Build history of the part. All positions in model axes, mm. Face numbers are marked on the shaded views. Round coordinates to 2 decimals unless told otherwise and drop trailing zeros. Loops run counter-clockwise (first coordinate to the right, second up) from the corner with the lowest first, then second, coordinate; pieces in that order, holes last. Notation, with made-up numbers: (23.25, -35) - (52.25, -35) arc R17 cw to (52.25, -9) - close; hole circle Ø5 at (36, -15.75). An arc over 180 degrees is marked (long way). Put each result on its own line as item: value. Start each with the question number.
from build123d import *

# Parameters (mm, degrees)
SKETCH1_W                      = 600
SKETCH1_H                      = 206.35
BASE_FLANGE1_DEPTH             = 3.18
SKETCH6_W                      = 25.4
SKETCH6_H                      = 6
CUT_EXTRUDE1_DEPTH             = 10
EDGE_FLANGE1_STRIP_W           = 14.1932
EDGE_FLANGE1_STRIP_H           = 3.18
EDGE_FLANGE1_STRIP_CUT_DEPTH   = 549.2
EDGE_FLANGE1_STRIP_2_W         = 14.1932
EDGE_FLANGE1_STRIP_2_H         = 3.18
EDGE_FLANGE1_STRIP_CUT_2_DEPTH = 549.2
EDGE_FLANGE1_DEPTH             = 549.2
EDGE_FLANGE1_BEND_DEPTH        = 549.2
SKETCH15_W                     = 498.4
SKETCH15_H                     = 171.408066666
CUT_EXTRUDE2_DEPTH             = 10
FILLET1_R                      = 5
SKETCH16_R                     = 1.65
CUT_EXTRUDE3_DEPTH             = 10
SKETCH17_R                     = 1.65
CUT_EXTRUDE4_DEPTH             = 366.000660958


# Sheet-metal steps are written as plain solids
with BuildPart() as part:
    # Sketch1 → Base-Flange1 (new body)
    with BuildSketch(Plane.XY):
        Rectangle(SKETCH1_W, SKETCH1_H)
    extrude(amount=-BASE_FLANGE1_DEPTH)

    # Sketch6 → Cut-Extrude1 (cut)
    with BuildSketch(Plane.XY):
        with Locations((-287.3, 100.175)):
            Rectangle(SKETCH6_W, SKETCH6_H)
        with Locations((-287.3, -100.175)):
            Rectangle(SKETCH6_W, SKETCH6_H)
        with Locations((287.3, -100.175)):
            Rectangle(SKETCH6_W, SKETCH6_H)
        with Locations((287.3, 100.175)):
            Rectangle(SKETCH6_W, SKETCH6_H)
    extrude(amount=-CUT_EXTRUDE1_DEPTH, mode=Mode.SUBTRACT)

    # Edge-Flange1 strip (across the edge) → Edge-Flange1 strip cut (cut)
    with BuildSketch(Plane(origin=(-274.6, 103.175, -3.18), x_dir=(0, -1, 0), z_dir=(1, 0, 0))):
        with Locations((-3.18, -1.59)):
            Rectangle(EDGE_FLANGE1_STRIP_W, EDGE_FLANGE1_STRIP_H)
    extrude(amount=EDGE_FLANGE1_STRIP_CUT_DEPTH, mode=Mode.SUBTRACT)

    # Edge-Flange1 strip 2 (across the edge) → Edge-Flange1 strip cut 2 (cut)
    with BuildSketch(Plane(origin=(274.6, -103.175, -3.18), x_dir=(0, 1, 0), z_dir=(-1, 0, 0))):
        with Locations((-3.18, -1.59)):
            Rectangle(EDGE_FLANGE1_STRIP_2_W, EDGE_FLANGE1_STRIP_2_H)
    extrude(amount=EDGE_FLANGE1_STRIP_CUT_2_DEPTH, mode=Mode.SUBTRACT)

    # Edge-Flange1 section (across the edge) → Edge-Flange1 (add)
    with BuildSketch(Plane(origin=(-274.6, 103.175, -3.18), x_dir=(0, -1, 0), z_dir=(1, 0, 0))):
        with BuildLine():
            Line((0, 0.7366), (0, 22.22))
            Line((0, 22.22), (3.18, 22.22))
            Line((3.18, 22.22), (3.18, 0.7366))
            ThreePointArc((3.18, 0.7366), (3.395745145, 0.215745145), (3.9166, 0))
            Line((3.9166, 0), (3.9166, -3.18))
            ThreePointArc((3.9166, -3.18), (1.147145581, -2.032854419), (0, 0.7366))
        make_face()
    extrude(amount=EDGE_FLANGE1_DEPTH)

    # Edge-Flange1 section 2 (across the edge) → Edge-Flange1 bend (add)
    with BuildSketch(Plane(origin=(274.6, -103.175, -3.18), x_dir=(0, 1, 0), z_dir=(-1, 0, 0))):
        with BuildLine():
            Line((0, 0.7366), (0, 22.22))
            Line((0, 22.22), (3.18, 22.22))
            Line((3.18, 22.22), (3.18, 0.7366))
            ThreePointArc((3.18, 0.7366), (3.395745145, 0.215745145), (3.9166, 0))
            Line((3.9166, 0), (3.9166, -3.18))
            ThreePointArc((3.9166, -3.18), (1.147145581, -2.032854419), (0, 0.7366))
        make_face()
    extrude(amount=EDGE_FLANGE1_BEND_DEPTH)

    # Sketch15 → Cut-Extrude2 (cut)
    with BuildSketch(Plane.XY):
        Rectangle(SKETCH15_W, SKETCH15_H)
    extrude(amount=-CUT_EXTRUDE2_DEPTH, mode=Mode.SUBTRACT)

    # Fillet1
    fillet1_edges = [part.edges().sort_by_distance(p)[0] for p in [
        (249.2, 85.704033333, -1.59),
        (249.2, -85.704033333, -1.59),
        (-249.2, -85.704033333, -1.59),
        (-249.2, 85.704033333, -1.59),
    ]]
    fillet(fillet1_edges, radius=FILLET1_R)

    # Sketch16 → Cut-Extrude3 (cut)
    with BuildSketch(Plane.XY):
        with Locations((-287.3, 0)):
            Circle(SKETCH16_R)
        with Locations((-287.3, 20)):
            Circle(SKETCH16_R)
        with Locations((-287.3, 40)):
            Circle(SKETCH16_R)
        with Locations((-287.3, 60)):
            Circle(SKETCH16_R)
        with Locations((-287.3, -20)):
            Circle(SKETCH16_R)
        with Locations((-287.3, -40)):
            Circle(SKETCH16_R)
        with Locations((-287.3, -60)):
            Circle(SKETCH16_R)
        with Locations((287.3, -60)):
            Circle(SKETCH16_R)
        with Locations((287.3, -40)):
            Circle(SKETCH16_R)
        with Locations((287.3, -20)):
            Circle(SKETCH16_R)
        with Locations((287.3, 0)):
            Circle(SKETCH16_R)
        with Locations((287.3, 20)):
            Circle(SKETCH16_R)
        with Locations((287.3, 40)):
            Circle(SKETCH16_R)
        with Locations((287.3, 60)):
            Circle(SKETCH16_R)
        with Locations((-287.3, 80)):
            Circle(SKETCH16_R)
        with Locations((-287.3, -80)):
            Circle(SKETCH16_R)
        with Locations((287.3, -80)):
            Circle(SKETCH16_R)
        with Locations((287.3, 80)):
            Circle(SKETCH16_R)
    extrude(amount=-CUT_EXTRUDE3_DEPTH, mode=Mode.SUBTRACT)

    # Sketch17 → Cut-Extrude4 (cut, through all)
    with BuildSketch(Plane(origin=(0, 103.175, 0), x_dir=(1, 0, 0), z_dir=(0, 1, 0))):
        with Locations(Location((0, 12.7, 0), (0, 0, 270))):
            Circle(SKETCH17_R)
        with Locations(Location((20, 12.7, 0), (0, 0, 270))):
            Circle(SKETCH17_R)
        with Locations(Location((40, 12.7, 0), (0, 0, 270))):
            Circle(SKETCH17_R)
        with Locations(Location((60, 12.7, 0), (0, 0, 270))):
            Circle(SKETCH17_R)
        with Locations(Location((80, 12.7, 0), (0, 0, 270))):
            Circle(SKETCH17_R)
        with Locations(Location((100, 12.7, 0), (0, 0, 270))):
            Circle(SKETCH17_R)
        with Locations(Location((120, 12.7, 0), (0, 0, 270))):
            Circle(SKETCH17_R)
        with Locations(Location((140, 12.7, 0), (0, 0, 270))):
            Circle(SKETCH17_R)
        with Locations(Location((160, 12.7, 0), (0, 0, 270))):
            Circle(SKETCH17_R)
        with Locations(Location((180, 12.7, 0), (0, 0, 270))):
            Circle(SKETCH17_R)
        with Locations(Location((200, 12.7, 0), (0, 0, 270))):
            Circle(SKETCH17_R)
        with Locations(Location((220, 12.7, 0), (0, 0, 270))):
            Circle(SKETCH17_R)
        with Locations(Location((240, 12.7, 0), (0, 0, 270))):
            Circle(SKETCH17_R)
        with Locations(Location((260, 12.7, 0), (0, 0, 270))):
            Circle(SKETCH17_R)
        with Locations(Location((-20, 12.7, 0), (0, 0, 270))):
            Circle(SKETCH17_R)
        with Locations(Location((-40, 12.7, 0), (0, 0, 270))):
            Circle(SKETCH17_R)
        with Locations(Location((-60, 12.7, 0), (0, 0, 270))):
            Circle(SKETCH17_R)
        with Locations(Location((-80, 12.7, 0), (0, 0, 270))):
            Circle(SKETCH17_R)
        with Locations(Location((-100, 12.7, 0), (0, 0, 270))):
            Circle(SKETCH17_R)
        with Locations(Location((-120, 12.7, 0), (0, 0, 270))):
            Circle(SKETCH17_R)
        with Locations(Location((-140, 12.7, 0), (0, 0, 270))):
            Circle(SKETCH17_R)
        with Locations(Location((-160, 12.7, 0), (0, 0, 270))):
            Circle(SKETCH17_R)
        with Locations(Location((-180, 12.7, 0), (0, 0, 270))):
            Circle(SKETCH17_R)
        with Locations(Location((-200, 12.7, 0), (0, 0, 270))):
            Circle(SKETCH17_R)
        with Locations(Location((-220, 12.7, 0), (0, 0, 270))):
            Circle(SKETCH17_R)
        with Locations(Location((-240, 12.7, 0), (0, 0, 270))):
            Circle(SKETCH17_R)
        with Locations(Location((-260, 12.7, 0), (0, 0, 270))):
            Circle(SKETCH17_R)
    extrude(amount=-CUT_EXTRUDE4_DEPTH, mode=Mode.SUBTRACT)


solid = part.part
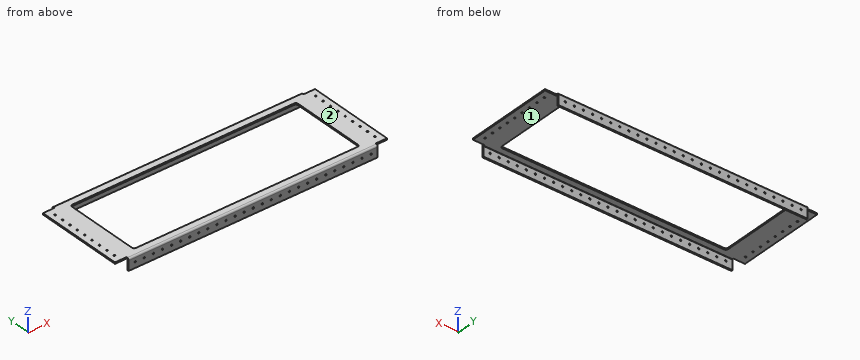
1) Drop flat-ended pins along their axis: pin 1 Ø6 at (x, z) = (-51.5, -3.5) entering from +Y (3 decimals); pin 2 Ø5.5 at (x, y) = (-287.3, 60) entering from -Z. Give the stop position or say it passes through.
2) Drill centre lines: line 1 (X direction, y = 80, z = -1.3); line 2 (Y direction, x = -87, z = -5) (3 decimals); line 3 (X direction, y = 2, z = -1.25). Where is each one in solid material? Low to high. Write a range as [from, to].
3) Slice it at A-A, the plane y = -72.5. Write the cut outline in (x, z), and give its area (3 significant figures).
4) Pull direction Y, two halves, no side cores. Call the marked faces 1 and 2: pulls with the +Y half, pulls with the -Y half, needs draft (parallel to the pull), parting line crosses it, or undercut.
Taken from the geometry:
1. pin 1: stops at y = 103.175
1. pin 2: stops at z = -3.18
2. line 1: x = [-300, -288.95], [-285.65, -249.2], [249.2, 285.65], [288.95, 300]
2. line 2: y = [-103.175, -99.995], [99.995, 103.175]
2. line 3: x = [-300, -249.2], [249.2, 300]
3. outline: (-300, -3.18) - (-249.2, -3.18) - (-249.2, 0) - (-300, 0) - close; (249.2, -3.18) - (300, -3.18) - (300, 0) - (249.2, 0) - close
3. area: 323 mm2
4. face 1: undercut
4. face 2: needs draft
